Check sheet for the drawn part. Datum: minimum x, y, z corner. Units: mm. A direction names the side the tool comes from. Coordinates: 2 decimals unless noted, no trailing zeros. Loops run counter-clockwise (first coordinate to the right, second up) from the corner with the lowest first, then second, coordinate; pieces in that order, holes last. Notation, with made-up numbers: (62, 58.5) - (82, 58.5) arc R23 cw to (82, 70.5) - close; hole circle Ø7 at (84.5, 19). An arc over 180 degrees is marked (long way). Write item = value, one per line. Start each with the question number.
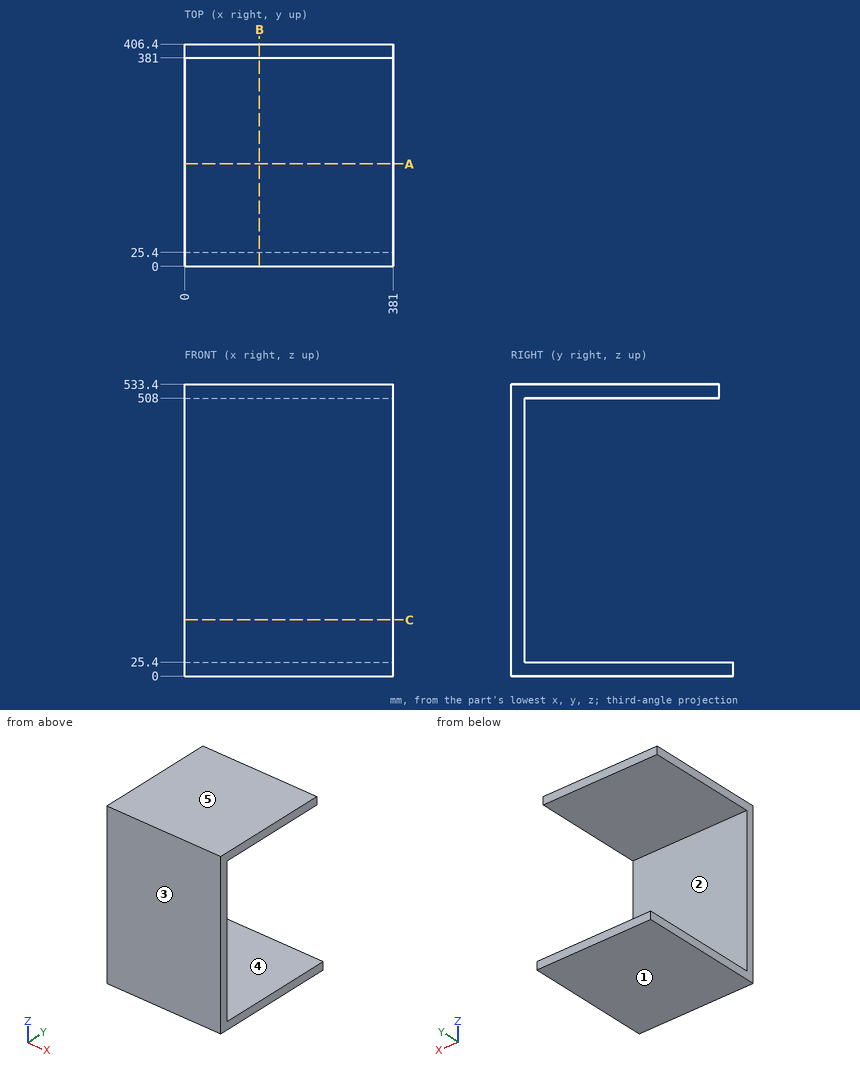
(1) Depth check by flat-ended pin: pin 1 (7.5 mm diameter, centred on x = 212.5, z = 516, fed in from +Y); pin 2 (12 mm diameter, centred on x = 181.5, z = 399.5, fed in from +Y). Enter the tip coordinate at first touch or a pass-through.
(2) Tool access check on the marked faces 4 and 5. Record the directions out of +Z, -Z, +X, -X, +Y, -Y that give a thin tool (end or side, any length) a straight path to the whole face; none if there is none.
(3) Scan lines: line 1 (Z direction, x = 189.5, y = 134); line 2 (Y direction, x = 260, z = 105). Record each from-to range of solid material in increasing order.
(4) Sectioned sample at A-A on y = 187. Enter the section's corners in (x, z).
(5) Sectioned sample at B-B on x = 136.5. Enter the section's corners in (y, z), plus the area to 3 significant figures.
(6) Draft check along Z on the marked faces 1, 2 and 3. Enter one of: pulls with the +Z half, pulls with the -Z half, needs draft (parallel to the pull), parting line crosses it, or undercut.
(7) Sectioned sample at C-C on z = 102.5. Enter the section's corners in (x, y), plus the area to 3 significant figures.
Working result:
q1.pin_1 = 381
q1.pin_2 = 25.4
q2.face_4 = +X, -X, +Y
q2.face_5 = +Z, +X, -X, +Y, -Y
q3.line_1 = 0 to 25.4, 508 to 533.4
q3.line_2 = 0 to 25.4
q4.outline = (0, 0) - (381, 0) - (381, 25.4) - (0, 25.4) - close; (0, 508) - (381, 508) - (381, 533.4) - (0, 533.4) - close
q5.outline = (0, 0) - (406.4, 0) - (406.4, 25.4) - (25.4, 25.4) - (25.4, 508) - (381, 508) - (381, 533.4) - (0, 533.4) - close
q5.area = 32,300 mm2
q6.face_1 = pulls with the -Z half
q6.face_2 = undercut
q6.face_3 = needs draft
q7.outline = (0, 0) - (381, 0) - (381, 25.4) - (0, 25.4) - close
q7.area = 9,680 mm2
